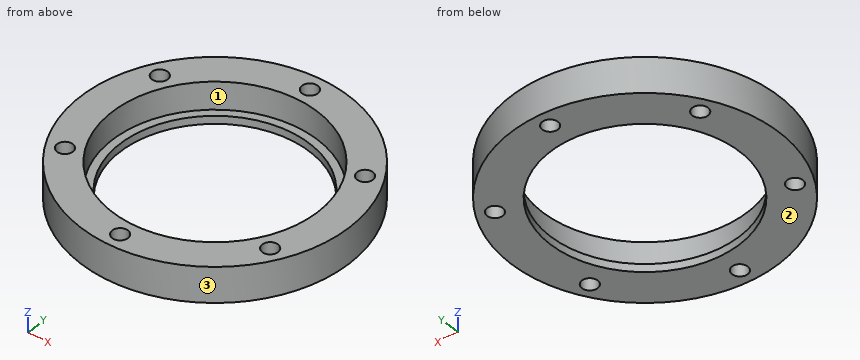
from build123d import *

# Parameters (mm, degrees)
SKETCH_1_R          = 34
EXTRUDE_1_DEPTH     = 9
SKETCH_2_R          = 26
CUT_EXTRUDE_1_DEPTH = 7
SKETCH_3_R          = 24
CUT_EXTRUDE_2_DEPTH = 8
SKETCH_4_R          = 2
CUT_EXTRUDE_3_DEPTH = 49.918299235


with BuildPart() as part:
    # 草图1 → 凸台-拉伸1 (new body)
    with BuildSketch(Plane.XY):
        Circle(SKETCH_1_R)
    extrude(amount=EXTRUDE_1_DEPTH)

    # 草图2 → 切除-拉伸1 (cut)
    with BuildSketch(Plane.XY.offset(9)):
        Circle(SKETCH_2_R)
    extrude(amount=-CUT_EXTRUDE_1_DEPTH, mode=Mode.SUBTRACT)

    # 草图3 → 切除-拉伸2 (cut)
    with BuildSketch(Plane.XY.offset(2)):
        Circle(SKETCH_3_R)
    extrude(amount=-CUT_EXTRUDE_2_DEPTH, mode=Mode.SUBTRACT)

    # 草图4 → 切除-拉伸3 (cut, through all)
    with BuildSketch(Plane.XY.offset(9)):
        with Locations((0, 30)):
            Circle(SKETCH_4_R)
        with Locations((25.980762114, 15)):
            Circle(SKETCH_4_R)
        with Locations((25.980762114, -15)):
            Circle(SKETCH_4_R)
        with Locations((0, -30)):
            Circle(SKETCH_4_R)
        with Locations((-25.980762114, -15)):
            Circle(SKETCH_4_R)
        with Locations((-25.980762114, 15)):
            Circle(SKETCH_4_R)
    extrude(amount=-CUT_EXTRUDE_3_DEPTH, mode=Mode.SUBTRACT)


solid = part.part
Build history of the part. All positions in model axes, mm. Face numbers are marked on the shaded views. Round coordinates to 2 decimals unless told otherwise and drop trailing zeros. Loops run counter-clockwise (first coordinate to the right, second up) from the corner with the lowest first, then second, coordinate; pieces in that order, holes last. Notation, with made-up numbers: (-34.5, 80.25) -> (-5.5, 80.25) arc R21 ccw to (-5.5, 98.25) -> close; hole circle Ø10 at (-35.5, 29.5). An arc over 180 degrees is marked (long way). One line per item, written item: value. Start each with the question number.
Q1. Two-plate mould, pull along X, no slides. Class the marked faces 1, 2 and 3: released by +X, released by -X, zero draft, split by the parting line, or undercut.
Q2. Cut at C-C on y = -30. List the corners of the cut face in (x, z), plus the area to 3 significant figures.
Q3. Probe line 1 along Y through (x, z) = (0, 1.5); line 2 along Y through (x, z) = (0, 3.5); line 3 along X through (y, z) = (-16, 2.25). List the from-to ranges inside material, lowest first.
Q4. Drop flat-ended pins along their axis: pin 1 Ø1 at (x, z) = (2.5, 8) entering from +Y; pin 2 Ø1 at (y, z) = (-15.5, 3.5) entering from +X; pin 3 Ø5 at (y, z) = (8.5, 2) entering from -X. Give the stop position or say it passes through.
Q5. Cut at B-B on x = 0. List the corners of the cut face in (y, z).
Q6. Cut at A-A on z = 6. List the corners of the cut face in (x, y).
Q7. Cut at D-D on y = 15. List the corners of the cut face in (x, z) (3 decimals).
Computed:
1. face 1: undercut
1. face 2: zero draft
1. face 3: split by the parting line
2. outline: (-16, 0) -> (-2, 0) -> (-2, 9) -> (-16, 9) -> close; (2, 0) -> (16, 0) -> (16, 9) -> (2, 9) -> close
2. area: 252 mm²
3. line 1: -34 to -32, -28 to -24, 24 to 28, 32 to 34
3. line 2: -34 to -32, -28 to -26, 26 to 28, 32 to 34
3. line 3: -30 to -27.71, -24.25 to -20.49, 20.49 to 24.25, 27.71 to 30
4. pin 1: y = 33.94
4. pin 2: x = 30.51
4. pin 3: x = -33.47
5. outline: (-34, 0) -> (-32, 0) -> (-32, 9) -> (-34, 9) -> close; (-28, 0) -> (-24, 0) -> (-24, 2) -> (-26, 2) -> (-26, 9) -> (-28, 9) -> close; (24, 0) -> (28, 0) -> (28, 9) -> (26, 9) -> (26, 2) -> (24, 2) -> close; (32, 0) -> (34, 0) -> (34, 9) -> (32, 9) -> close
6. outline: circle Ø68 at (0, 0); hole circle Ø4 at (-25.98, -15); hole circle Ø4 at (-25.98, 15); hole circle Ø52 at (0, 0); hole circle Ø4 at (0, -30); hole circle Ø4 at (0, 30); hole circle Ø4 at (25.98, -15); hole circle Ø4 at (25.98, 15)
7. outline: (-30.512, 0) -> (-27.981, 0) -> (-27.981, 9) -> (-30.512, 9) -> close; (-23.981, 0) -> (-18.735, 0) -> (-18.735, 2) -> (-21.237, 2) -> (-21.237, 9) -> (-23.981, 9) -> close; (18.735, 0) -> (23.981, 0) -> (23.981, 9) -> (21.237, 9) -> (21.237, 2) -> (18.735, 2) -> close; (27.981, 0) -> (30.512, 0) -> (30.512, 9) -> (27.981, 9) -> close
